Input: dimensioned drawing with shaded views. Units: mm. Origin: part minimum x, y, z. A direction names the side the tool comes from. Give positions to 0.01 mm unless a question says otherwise; leave off trailing zeros. Write each loop counter-clockwise with the first axis right and the second up, starting at its lowest first coordinate (ties: lowest second). Pieces come first, ordered by that corner, then holes. Notation, with made-up numbers: (53, -31) - (67, -31) arc R34 ccw to (67, -1) - close; hole circle Ø11 at (-14.75, 59). An arc over 180 degrees is marked (long way). Answer as CSV lines item,"result".
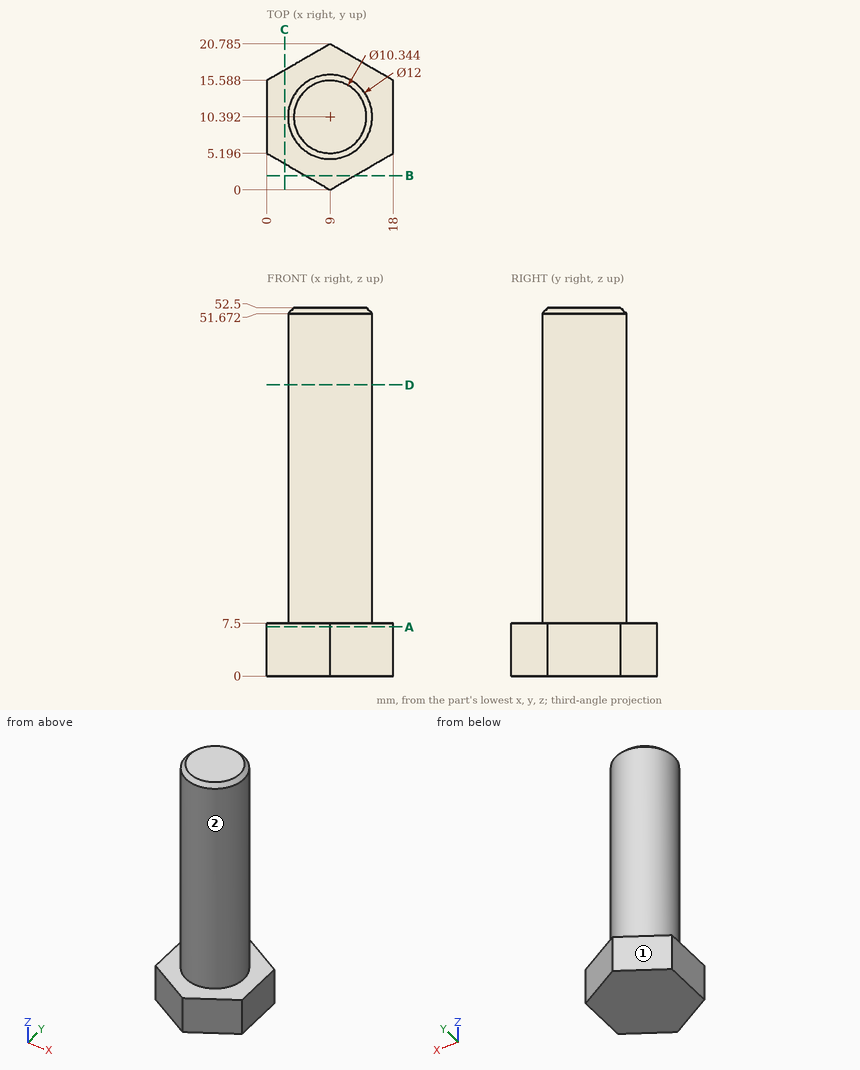
Item 1: Cut plane D-D on z = 41.5. Return the cut outline in (x, y), plus the area to 3 significant figures.
The answers:
outline,"circle Ø12 at (9, 10.39)"
area,"113 mm²"
Item 2: Contact query for flat-ended pins moving along their axis: pin 1 (5 mm diameter, centred on y = 6, z = 28, fed in from -X); pin 2 (4 mm diameter, centred on y = 5, z = 38.5, fed in from +X); pin 3 (5 mm diameter, centred on x = 8.5, y = 17.5, fed in from +Z); pin 4 (4 mm diameter, centred on x = 7.5, z = 24.5, fed in from +Y). Output: stop coordinate, or through.
The answers:
pin 1,"x = 3.31"
pin 2,"x = 13.95"
pin 3,"z = 52.5"
pin 4,"y = 16.39"
Item 3: Cut plane B-B on y = 2. Return the cut outline in (x, z) (1 decimal).
The answers:
outline,"(5.5, 0) - (12.5, 0) - (12.5, 7.5) - (5.5, 7.5) - close"
Item 4: Ray query, line 1 (Z direction, x = 3.25, y = 8); line 2 (Y direction, x = 9, z = 50.5); line 3 (Y direction, x = 13.25, z = 34) (1 decimal). Return the intervals inside material, ascending. Write a range as from..to.
The answers:
line 1,"0..7.5"
line 2,"4.39..16.39"
line 3,"6.2..14.6"
Item 5: Cut plane C-C on x = 2.5. Return the cut outline in (y, z).
The answers:
outline,"(3.75, 0) - (17.03, 0) - (17.03, 7.5) - (3.75, 7.5) - close"
Item 6: Reachability of the marked faces 1 and 2 from +Z, -Z, +X, -X, +Y, -Y: full face, straight path, thin tool, end or side. Return the list, or none.
The answers:
face 1,"+Z, -Z, -X, +Y"
face 2,"+Z"
Item 7: Cut plane A-A on z = 7. Return the cut outline in (x, y) (1 decimal).
The answers:
outline,"(0, 5.2) - (9, 0) - (18, 5.2) - (18, 15.6) - (9, 20.8) - (0, 15.6) - close"
